Autodesk Inventor part; units mm, degrees
ref_plane "YZ Plane" through (0, 0, 0) normal (1, 0, 0) x (0, 1, 0)
ref_plane "XZ Plane" through (0, 0, 0) normal (0, 1, 0) x (-1, 0, 0)
ref_plane "XY Plane" through (0, 0, 0) normal (0, 0, 1) x (1, 0, 0)
sketch "Sketch1" plane through (0, 0, 0) normal (0, 1, 0) x (-1, 0, 0)
  line L0 (0, 0) -> (40, 0)
  line L1 (40, 0) -> (40, -40)
  line L2 (40, -40) -> (0, -40)
  line L3 (0, -40) -> (0, 0)
  line L4 (40, 0) -> (80, 0)
  line L5 (80, 0) -> (80, -80)
  line L6 (80, -80) -> (40, -80)
  line L7 (40, -80) -> (40, 0)
  dimension "d0" = 40
  dimension "d1" = 40
  dimension "d2" = 40
  dimension "d3" = 80
extrude "Extrusion1" add sketch "Sketch1" along normal blind 6
sketch "Sketch2" plane through (0, 6, 0) normal (0, 1, 0) x (1, 0, 0)
  line L0 (0, 0) -> (0, 40)
  line L1 (0, 0) -> (0, 10)
  line L2 (0, 40) -> (0, 30)
  circle A0 centre (-10, 10) radius 2.75
  line L3 (-80, 0) -> (0, 0)
  circle A1 centre (-22, 10) radius 2.75
  circle A2 centre (-34, 10) radius 2.75
  circle A3 centre (-10, 30) radius 2.75
  circle A4 centre (-22, 30) radius 2.75
  circle A5 centre (-34, 30) radius 2.75
  circle A6 centre (-70, 70) radius 2.75
  line L4 (-80, 80) -> (-80, 0)
  line L5 (-40, 80) -> (-80, 80)
  circle A7 centre (-70, 50) radius 2.75
  circle A8 centre (-70, 30) radius 2.75
  circle A9 centre (-70, 10) radius 2.75
  circle A10 centre (-50, 70) radius 2.75
  circle A11 centre (-50, 50) radius 2.75
  circle A12 centre (-50, 30) radius 2.75
  circle A13 centre (-50, 10) radius 2.75
  dimension "d6" = 10
  dimension "d7" = 10
  dimension "d8" = 5.5
  dimension "d9" = 10
  dimension "d10" = 10
  dimension "d13" = 12
  dimension "d16" = 20
  dimension "d19" = 5.5
  dimension "d20" = 10
  dimension "d21" = 10
  dimension "d24" = 20
  dimension "d27" = 20
extrude "Extrusion2" cut sketch "Sketch2" against normal up to next
fillet "Fillet1" radius 2 6 edges at (0, 3, 0) (0, 3, -40) (-40, 3, -80) (-80, 3, 0) (-80, 3, -80) (-40, 3, -40)
properties part number "90deg_4040Bracket"
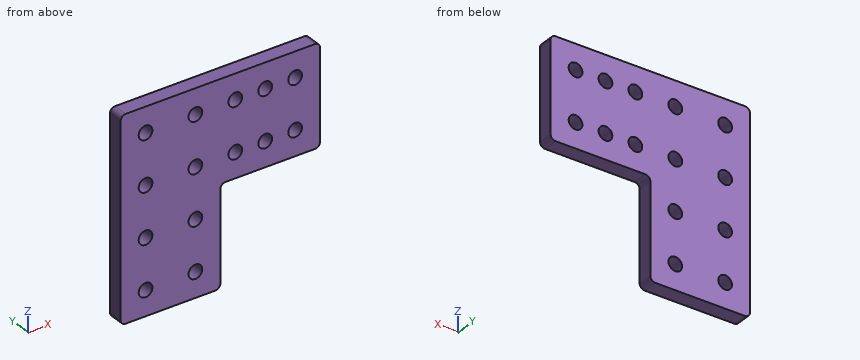
Could you check a few things on this model? Use its own coordinates, in mm. Give positions to 0.01 mm unless a question says otherwise; leave off trailing zeros. Loops run counter-clockwise (first coordinate to the right, second up) from the corner with the lowest first, then second, coordinate; pieces in that order, holes last. Notation, with made-up numbers: (11, 21.25) - (58, 21.25) arc R31 cw to (58, 45.25) - close; hole circle Ø9 at (82, 37.5). An arc over 180 degrees is marked (long way). Use one line per item in the form item = value.
1. I need wall thicknesses on probe 1 along Z at (x, y) = (-22, 1.95); probe 2 along X at (y, z) = (3.7, -10); probe 3 along Z at (x, y) = (-50, 2.55). Which ranges of each line are inside material? Lowest first, please.
Response values:
probe_1 = -40 to -32.75, -27.25 to -12.75, -7.25 to 0
probe_2 = -80 to -72.75, -67.25 to -52.75, -47.25 to -36.75, -31.25 to -24.75, -19.25 to -12.75, -7.25 to 0
probe_3 = -80 to -72.75, -67.25 to -52.75, -47.25 to -32.75, -27.25 to -12.75, -7.25 to 0
2. I'm going to push flat-ended pins straight in: pin 1 Ø4.5 at (x, z) = (-22, -30) entering from +Y; pin 2 Ø9 at (x, z) = (-10, -30) entering from +Y; pin 3 Ø2 at (x, y) = (-18, 4) entering from -Z. Where does each tip first touch, or does it pass through?
Response values:
pin_1 = through
pin_2 = 6
pin_3 = -40
3. I want a section at C-C (y = 3.8). Give the number of separate pieces and of enclosed holes in the cut face, and give its area (3 significant figures).
Response values:
separate_pieces = 1
enclosed_holes = 14
area = 4,460 mm²
4. I want a section at B-B (z = -50). Please give me the cut outline in (x, y).
Response values:
outline = (-80, 0) - (-72.75, 0) - (-72.75, 6) - (-80, 6) - close; (-67.25, 0) - (-52.75, 0) - (-52.75, 6) - (-67.25, 6) - close; (-47.25, 0) - (-40, 0) - (-40, 6) - (-47.25, 6) - close
5. I want a section at D-D (x = -21.5). Please give me the cut outline in (y, z), and give its area (3 significant figures).
Response values:
outline = (0, -40) - (6, -40) - (6, -32.7) - (0, -32.7) - close; (0, -27.3) - (6, -27.3) - (6, -12.7) - (0, -12.7) - close; (0, -7.3) - (6, -7.3) - (6, 0) - (0, 0) - close
area = 175 mm²
6. I want a section at A-A (x = -70). Please give me the cut outline in (y, z), and give its area (3 significant figures).
Response values:
outline = (0, -80) - (6, -80) - (6, -72.75) - (0, -72.75) - close; (0, -67.25) - (6, -67.25) - (6, -52.75) - (0, -52.75) - close; (0, -47.25) - (6, -47.25) - (6, -32.75) - (0, -32.75) - close; (0, -27.25) - (6, -27.25) - (6, -12.75) - (0, -12.75) - close; (0, -7.25) - (6, -7.25) - (6, 0) - (0, 0) - close
area = 348 mm²
